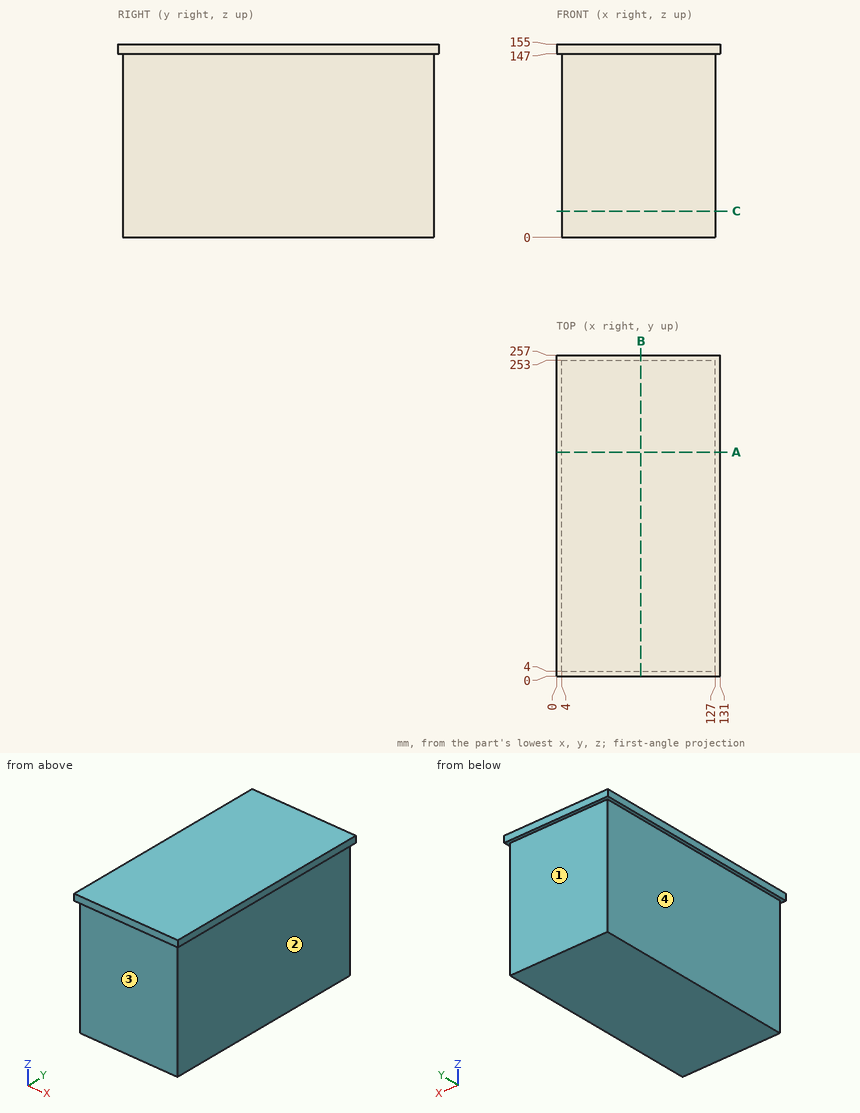
The drawing under review shows one solid part. Ordinate dimensions are in mm from its lowest x, y, z. A direction names the side the tool comes from. Round coordinates to 2 decimals unless told otherwise and drop trailing zeros. Loops run counter-clockwise (first coordinate to the right, second up) from the corner with the lowest first, then second, coordinate; pieces in that order, holes last. Notation, with made-up numbers: (29.25, -27) -> (59.25, -27) arc R19 ccw to (59.25, 8) -> close; hole circle Ø9 at (6.25, 20). An arc over 180 degrees is marked (long way). Answer in a Markdown table with one row per item.
1) Consider section A-A, the plane y = 179.5. Write out the cut boundary in (x, z).
Taken from the geometry:
| item | result |
|---|---|
| outline | (0, 147) -> (4, 147) -> (4, 0) -> (127, 0) -> (127, 147) -> (131, 147) -> (131, 155) -> (0, 155) -> close |
2) Consider section B-B, the plane x = 67.5. Write out the cut boundary in (y, z), plus the area to 3 significant figures.
Taken from the geometry:
| item | result |
|---|---|
| outline | (0, 147) -> (4, 147) -> (4, 0) -> (253, 0) -> (253, 147) -> (257, 147) -> (257, 155) -> (0, 155) -> close |
| area | 38,700 mm² |
3) For pin 1 Ø10 at (x, z) = (89, 35.5) entering from -Y; pin 2 Ø5 at (y, z) = (41, 42.5) entering from +X; pin 3 Ø1.5 at (x, z) = (48, 104) entering from +Y; pin 4 Ø1 at (x, y) = (53, 192.5) entering from -Z, all flat-tipped, find the tip position at first contact; note any pin that passes through.
Taken from the geometry:
| item | result |
|---|---|
| pin 1 | stops at y = 4 |
| pin 2 | stops at x = 127 |
| pin 3 | stops at y = 253 |
| pin 4 | stops at z = 0 |
4) Wall thickness on line 1 along Y through (x, z) = (40.5, 26.5); line 2 along X through (y, z) = (118, 88.5): over which ranges is each line inside the solid? List them lowest first.
Taken from the geometry:
| item | result |
|---|---|
| line 1 | y = 4 to 253 |
| line 2 | x = 4 to 127 |
5) Tool access review of the marked faces 1, 2, 3 and 4: name each direction out of +Z, -Z, +X, -X, +Y, -Y from which nothing blocks a thin tool from reaching the whole face with its end or side.
Taken from the geometry:
| item | result |
|---|---|
| face 1 | -Z, +X, -X, +Y |
| face 2 | -Z, +X, +Y, -Y |
| face 3 | -Z, +X, -X, -Y |
| face 4 | -Z, -X, +Y, -Y |
6) Consider section C-C, the plane z = 21. Write out the cut boundary in (x, y).
Taken from the geometry:
| item | result |
|---|---|
| outline | (4, 4) -> (127, 4) -> (127, 253) -> (4, 253) -> close |
